Part model, mm, in its own coordinate system. A direction names the side the tool comes from. Round coordinates to 2 decimals unless told otherwise and drop trailing zeros. Order: outer loops, then holes, each group sorted by start corner. A loop starts at its lowest first (then second) coordinate and runs counter-clockwise, first axis right, second up. Notation, with made-up numbers: (85, 63.25) - (140, 63.25) arc R11 cw to (140, 74.25) - close; hole circle Ø1 at (78.5, 28). An arc over 180 degrees is marked (long way). Return JSON: item names as keys, results as strings. Group by question number.
Item 1: Saw through at A-A on y = 150. List the corners of the cut face in (x, z), and give its area (3 significant figures).
Item 2: Saw through at B-B on x = 192. List the corners of the cut face in (y, z), and give its area (3 significant figures).
Item 3: Two-plate mould, pull along X, no slides. Class faces 1 (the face through (-258.05, 208.53, 2.46)), 2 (the face through (145.52, 11.86, 2.46)), 3 (the face through (1, 155, 0)): released by +X, released by -X, zero draft, split by the parting line, or undercut.
Item 4: Drop flat-ended pins along their axis: pin 1 (3 mm diameter, centred on y = 121.5, z = 3, fed in from -X); pin 2 (2.5 mm diameter, centred on x = -51, z = 2.5, fed in from -Y); pin 3 (3 mm diameter, centred on x = 185, z = 4, fed in from +Y). Give the stop position or say it passes through.
Item 5: Saw through at D-D on y = 103.5. List the corners of the cut face in (x, z).
Item 6: Tool access for faces 4 (the face through (27.78, 241.17, 2.46)), 5 (the face through (184.383, 269.744, 2.465)): list every direction of +Z, -Z, +X, -X, +Y, -Y with a clear straight run to the whole face (end or side of a thin tool).
Item 7: Probe probe 1 along X at (y, z) = (150, 1.3); probe 2 along X at (y, z) = (63.5, 2.05); probe 3 along X at (y, z) = (245, 2.95). List the from-to ranges inside material, lowest first.
```python
from build123d import *

# Parameters (mm, degrees)
PAD_DEPTH = 5


with BuildPart() as part:
    # Sketch → Pad (new body)
    with BuildSketch(Plane.XY):
        with BuildLine():
            ThreePointArc((136.38997, 21), (179.654002, 271.532264), (54.907669, 50))
            Line((52.707669, 50), (54.907669, 50))
            Line((52.707669, 44), (52.707669, 50))
            Line((50.507669, 44), (52.707669, 44))
            Line((50.507669, 50), (50.507669, 44))
            Line((-50.507669, 50), (50.507669, 50))
            Line((-50.507669, 44), (-50.507669, 50))
            Line((-52.707669, 44), (-50.507669, 44))
            Line((-52.707669, 50), (-52.707669, 44))
            Line((-54.907669, 50), (-52.707669, 50))
            ThreePointArc((-54.907669, 50), (-179.654002, 271.532264), (-136.38997, 21))
            Line((-136.38997, 21), (-136.38997, 18.7))
            Line((-136.38997, 18.7), (-130.38997, 18.7))
            Line((-130.38997, 18.7), (-130.38997, 16.5))
            Line((-130.38997, 16.5), (-136.38997, 16.5))
            Line((-136.38997, 16.5), (-136.38997, 2.000139))
            ThreePointArc((-136.38997, 2.000139), (-145.370032, 11.755646), (-157.678116, 16.687428))
            ThreePointArc((-50.75348, 254.353599), (-259.514276, 205.388401), (-157.678116, 16.687428))
            ThreePointArc((-50.75348, 254.353599), (-28.126193, 241.300075), (-2.5, 236.231852))
            Line((-2.5, 216.231852), (-2.5, 236.231852))
            Line((2.5, 216.231852), (-2.5, 216.231852))
            Line((2.5, 236.231852), (2.5, 216.231852))
            ThreePointArc((2.5, 236.231852), (28.126198, 241.300076), (50.753488, 254.353606))
            ThreePointArc((157.678116, 16.687428), (259.514278, 205.388396), (50.753488, 254.353606))
            ThreePointArc((157.678116, 16.687428), (145.370032, 11.755646), (136.38997, 2.000139))
            Line((136.38997, 16.5), (136.38997, 2.000139))
            Line((130.38997, 16.5), (136.38997, 16.5))
            Line((130.38997, 18.7), (130.38997, 16.5))
            Line((136.38997, 18.7), (130.38997, 18.7))
            Line((136.38997, 21), (136.38997, 18.7))
        make_face()
    extrude(amount=PAD_DEPTH)


solid = part.part
```
Filled in:
{
 "1": {"outline": "(-271.4, 0) - (-265.4, 0) - (-265.4, 5) - (-271.4, 5) - close; (-7.4, 0) - (7.4, 0) - (7.4, 5) - (-7.4, 5) - close; (265.4, 0) - (271.4, 0) - (271.4, 5) - (265.4, 5) - close", "area": "134 mm^2"},
 "2": {"outline": "(26.98, 0) - (33.6, 0) - (33.6, 5) - (26.98, 5) - close; (266.4, 0) - (273.02, 0) - (273.02, 5) - (266.4, 5) - close", "area": "66.2 mm^2"},
 "3": {"face 1": "undercut", "face 2": "released by +X", "face 3": "zero draft"},
 "4": {"pin 1": "stops at x = -268.67", "pin 2": "stops at y = 44", "pin 3": "stops at y = 276.52"},
 "5": {"outline": "(-263.14, 0) - (-256.73, 0) - (-256.73, 5) - (-263.14, 5) - close; (-16.07, 0) - (16.07, 0) - (16.07, 5) - (-16.07, 5) - close; (256.73, 0) - (263.14, 0) - (263.14, 5) - (256.73, 5) - close"},
 "6": {"face 4": "+Z, -Z, +Y", "face 5": "+Z, -Z"},
 "7": {"probe 1": "x = -271.4 to -265.4, -7.4 to 7.4, 265.4 to 271.4", "probe 2": "x = -240.05 to -232.1, -40.7 to 40.7, 232.1 to 240.05", "probe 3": "x = -232.32 to -223.67, -49.13 to -36.49, 36.49 to 49.13, 223.67 to 232.32"}
}
